CAD build for the part. Positions are in the model's coordinates, mm. Give positions to 0.01 mm unless a question says otherwise; leave off trailing zeros. Order: outer loops, then holes, each group sorted by start corner. A loop starts at its lowest first (then second) coordinate and runs counter-clockwise, first axis right, second up.
from build123d import *

# Parameters (mm, degrees)
ESQUISSE1_R             = 65
BOSS_EXTRU_1_DEPTH      = 3
ESQUISSE2_R             = 1
ENL_V_MAT_EXTRU_1_DEPTH = 3
ESQUISSE3_R             = 7
ENL_V_MAT_EXTRU_2_DEPTH = 3
ESQUISSE4_R             = 1.5
ENL_V_MAT_EXTRU_4_DEPTH = 4


with BuildPart() as part:
    # Esquisse1 → Boss.-Extru.1 (new body)
    with BuildSketch(Plane(origin=(0, 0, 0), x_dir=(1, 0, 0), z_dir=(0, 1, 0))):
        with Locations(Location((0, 0, 0), (0, 0, 270))):
            Circle(ESQUISSE1_R)
    extrude(amount=BOSS_EXTRU_1_DEPTH)

    # Esquisse2 → Enlèv. mat.-Extru.1 (cut)
    with BuildSketch(Plane(origin=(0, 3, 0), x_dir=(1, 0, 0), z_dir=(0, 1, 0))):
        with Locations(Location((-53.47585562, 32.350932996, 0), (0, 0, 270))):
            Circle(ESQUISSE2_R)
        with Locations(Location((-54.754657621, -30.135982958, 0), (0, 0, 270))):
            Circle(ESQUISSE2_R)
        with Locations(Location((-1.278802001, -62.486915954, 0), (0, 0, 270))):
            Circle(ESQUISSE2_R)
        with Locations(Location((53.47585562, -32.350932996, 0), (0, 0, 270))):
            Circle(ESQUISSE2_R)
        with Locations(Location((54.754657621, 30.135982958, 0), (0, 0, 270))):
            Circle(ESQUISSE2_R)
        with Locations(Location((1.278802001, 62.486915954, 0), (0, 0, 270))):
            Circle(ESQUISSE2_R)
    extrude(amount=-ENL_V_MAT_EXTRU_1_DEPTH, mode=Mode.SUBTRACT)

    # Esquisse3 → Enlèv. mat.-Extru.2 (cut)
    with BuildSketch(Plane(origin=(0, 3, 0), x_dir=(1, 0, 0), z_dir=(0, 1, 0))):
        with Locations(Location((0, 0, 0), (0, 0, 270))):
            Circle(ESQUISSE3_R)
    extrude(amount=-ENL_V_MAT_EXTRU_2_DEPTH, mode=Mode.SUBTRACT)

    # Esquisse4 → Enlèv. mat.-Extru.4 (cut)
    with BuildSketch(Plane(origin=(0, 3, 0), x_dir=(1, 0, 0), z_dir=(0, 1, 0))):
        with Locations(Location((0, 33.5, 0), (0, 0, 270))):
            Circle(ESQUISSE4_R)
        with Locations(Location((29.011851027, 16.75, 0), (0, 0, 270))):
            Circle(ESQUISSE4_R)
        with Locations(Location((29.011851027, -16.75, 0), (0, 0, 270))):
            Circle(ESQUISSE4_R)
        with Locations(Location((0, -33.5, 0), (0, 0, 270))):
            Circle(ESQUISSE4_R)
        with Locations(Location((-29.011851027, -16.75, 0), (0, 0, 270))):
            Circle(ESQUISSE4_R)
        with Locations(Location((-29.011851027, 16.75, 0), (0, 0, 270))):
            Circle(ESQUISSE4_R)
    extrude(amount=-ENL_V_MAT_EXTRU_4_DEPTH, mode=Mode.SUBTRACT)


solid = part.part
1. Pin check, flat tips, straight feed: P1, Ø1.8, axis at x = 0, z = -33.5, coming from the -Y side; P2, Ø1.5, axis at x = 9, y = 2.5, coming from the -Z side. Stop position of each tip, or through.
2. Saw through at D-D on x = -46.5. Give the cut face in (y, z), plus the area to 3 significant figures.
3. Mould opens along Z. For faces 1 (the flat face through (1, 0, 14)), 2 (the cylindrical face through (-29.925, 1.521, 15.56)), 3 (the cylindrical face through (19.52, 1.48, 62)) say: released by +Z, released by -Z, zero draft, split by the parting line, or undercut.
4. Saw through at C-C on y = 0.6. State how many separate pieces and enclosed holes the cut face has, plus the area to 3 significant figures.
5. Saw through at B-B on z = 16.75. Give the cut face in (x, y), plus the area to 3 significant figures.
6. Saw through at A-A on z = 0. Give the cut face in (x, y), plus the area to 3 significant figures.
7. Wall check: line 1 (X direction, y = 1.3, z = -16.75); line 2 (Z direction, x = 2.5, y = 1.4); line 3 (X direction, y = 2, z = -31). Give the ranges that are in metal, low to high.
Reported:
1. P1: passes through
1. P2: stops at z = -64.47
2. outline: (0, -45.42) - (3, -45.42) - (3, 45.42) - (0, 45.42) - close
2. area: 273 mm2
3. face 1: zero draft
3. face 2: undercut
3. face 3: split by the parting line
4. separate pieces: 1
4. enclosed holes: 13
4. area: 13,100 mm2
5. outline: (-62.8, 0) - (-30.51, 0) - (-30.51, 3) - (-62.8, 3) - close; (-27.51, 0) - (27.51, 0) - (27.51, 3) - (-27.51, 3) - close; (30.51, 0) - (62.8, 0) - (62.8, 3) - (30.51, 3) - close
5. area: 359 mm2
6. outline: (-65, 0) - (-7, 0) - (-7, 3) - (-65, 3) - close; (7, 0) - (65, 0) - (65, 3) - (7, 3) - close
6. area: 348 mm2
7. line 1: x = -62.8 to -30.51, -27.51 to 27.51, 30.51 to 62.8
7. line 2: z = -64.95 to -6.54, 6.54 to 64.95
7. line 3: x = -57.13 to 54.25, 55.26 to 57.13
